Source: CAD feature listing. Evaluate the final solid. Frame: model axes, mm. A direction names the side the tool comes from. Round coordinates to 2 decimals unless told otherwise and drop trailing zeros. Order: outer loops, then holes, each group sorted by start corner. A loop starts at its lowest first (then second) coordinate and runs counter-clockwise, first axis right, second up. Notation, with made-up numbers: (18, -36.75) -> (68, -36.75) arc R14 cw to (68, -11.75) -> close; hole circle Ø4 at (-13.75, 8.5). An arc over 180 degrees is marked (long way). One line per item, written item: value. Start each with the question number.
1) Section C-C (z = 0). Return the cut outline in (x, y).
2) Reachability of faces 5 (the face through (-7.5, 0, 0)), 6 (the face through (-5, 2.25, 1)), 7 (the face through (20, 0, -19)) from +Z, -Z, +X, -X, +Y, -Y: full face, straight path, thin tool, end or side. Return the list, or none.
3) Section B-B (x = 0). Return the cut outline in (y, z), and give its area (3 significant figures).
4) Ray query, L1, parallel to X at y = -3, z = -3.25; L2, parallel to Z at x = 0, y = 4.85; L3, parallel to X at y = -2, z = -8. Return the intervals inside material, ascending.
5) Section A-A (y = -5). Return the cut outline in (x, z), and give its area (3 significant figures).
6) Mould query, pull axis X, two halves, no side actions, for faces 1 (the face through (-5, -2.25, 1)), 2 (the face through (-6.2, 0.1, 3)), 3 (the face through (0, 0, 5)), 4 (the face through (-20, 0, -19)). Classes: pulls with the +X half, pulls with the -X half, needs draft (parallel to the pull), parting line crosses it, or undercut.
7) Section D-D (y = 1). Return the cut outline in (x, z).
8) Pin query (flat end, axial travel): P1, Ø9, axis at x = 0, z = 0, coming from the -Y side; P2, Ø1.8, axis at y = 2, z = -10.5, coming from the -X side; P3, Ø5, axis at y = -4.5, z = 2, coming from the -X side; P4, Ø6.5, axis at y = 3, z = -10.5, coming from the +X side. Return the tip coordinate at first contact, or that it passes through.
```python
from build123d import *

# Parameters (mm, degrees)
SKETCH1_R                = 4
BOSS_EXTRUDE1_DEPTH      = 6
BOSS_EXTRUDE1_DEPTH_BACK = 6
CUT_EXTRUDE1_REACH       = 25
SKETCH2_W                = 1.5
SKETCH2_H                = 4.5


with BuildPart() as part:
    # Sketch1 → Boss-Extrude1 (new body, two sides)
    with BuildSketch(Plane(origin=(0, 0, 0), x_dir=(1, 0, 0), z_dir=(0, 1, 0))) as boss_extrude1_sk:
        with BuildLine():
            Line((-7.5, 3), (-7.5, -3))
            Line((-7.5, -3), (-4, -3))
            ThreePointArc((-4, -3), (-0.01892542, -4.999964183), (3.977175044, -3.030194493))
            Line((3.977175044, -3.030194493), (20, 18))
            Line((20, 18), (20, 20))
            Line((20, 20), (-20, 20))
            Line((-20, 20), (-20, 18))
            Line((-20, 18), (-7.5, 3))
        make_face()
        Circle(SKETCH1_R, mode=Mode.SUBTRACT)
        with BuildLine():
            Line((-18.047437581, 18), (-1, 18))
            Line((-1, 18), (-1, 4.898979486))
            ThreePointArc((-1, 4.898979486), (-3.189184695, 3.850857175), (-4.626858427, 1.895305015))
            Line((-4.626858427, 1.895305015), (-18.047437581, 18))
        make_face(mode=Mode.SUBTRACT)
        with BuildLine():
            Line((1, 4.898979486), (1, 18))
            Line((1, 18), (18.114239399, 18))
            Line((18.114239399, 18), (4.948014241, 0.719134947))
            ThreePointArc((4.948014241, 0.719134947), (3.634899372, 3.433293835), (1, 4.898979486))
        make_face(mode=Mode.SUBTRACT)
    extrude(amount=BOSS_EXTRUDE1_DEPTH)
    extrude(boss_extrude1_sk.sketch, amount=-BOSS_EXTRUDE1_DEPTH_BACK)

    # Sketch2 → Cut-Extrude1 (cut, up to next)
    with BuildSketch(Plane(origin=(0, 0, 3), x_dir=(-1, 0, 0), z_dir=(0, 0, -1)), mode=Mode.PRIVATE) as cut_extrude1_sk1:
        with Locations((5.15, 0)):
            Rectangle(SKETCH2_W, SKETCH2_H)
    cut_extrude1_tool1 = extrude(cut_extrude1_sk1.sketch, amount=CUT_EXTRUDE1_REACH, mode=Mode.PRIVATE) & part.part
    add(cut_extrude1_tool1.solids().sort_by_distance((-5.15, 0, 3))[0], mode=Mode.SUBTRACT)


solid = part.part
```
Findings:
1. outline: (-7.5, -6) -> (-4, -6) -> (-4, 6) -> (-7.5, 6) -> close; (4, -6) -> (6.29, -6) -> (6.29, 6) -> (4, 6) -> close; hole (-5.9, -2.25) -> (-4.4, -2.25) -> (-4.4, 2.25) -> (-5.9, 2.25) -> close
2. face 5: +Z, -X, +Y, -Y
2. face 6: +Z
2. face 7: +Z, -Z, +X, +Y, -Y
3. outline: (-6, -20) -> (6, -20) -> (6, -4) -> (-6, -4) -> close; (-6, 4) -> (6, 4) -> (6, 5) -> (-6, 5) -> close
3. area: 204 mm2
4. L1: -7.71 to -5.76, -3.8 to -2.33, 2.33 to 3.8, 6.88 to 8.76
4. L2: -20 to -4, 4 to 5
4. L3: -11.67 to -9.71, -1 to 1, 10.5 to 12.38
5. outline: (-20, -20) -> (20, -20) -> (20, -18) -> (3.98, 3.03) arc R5 ccw to (-4, 3) -> (-7.5, 3) -> (-7.5, -3) -> (-20, -18) -> close; hole (-18.05, -18) -> (-1, -18) -> (-1, -4.9) arc R5 cw to (-4.63, -1.9) -> close; hole circle Ø8 at (0, 0); hole (1, -18) -> (18.11, -18) -> (4.95, -0.72) arc R5 cw to (1, -4.9) -> close
5. area: 215 mm2
6. face 1: undercut
6. face 2: needs draft
6. face 3: parting line crosses it
6. face 4: pulls with the -X half
7. outline: (-20, -20) -> (20, -20) -> (20, -18) -> (3.98, 3.03) arc R5 ccw to (-4, 3) -> (-4.4, 3) -> (-4.4, -2.37) arc R5 ccw to (-1, -4.9) -> (-1, -18) -> (-18.05, -18) -> (-5.9, -3.42) -> (-5.9, 3) -> (-7.5, 3) -> (-7.5, -3) -> (-20, -18) -> close; hole circle Ø8 at (0, 0); hole (1, -18) -> (18.11, -18) -> (4.95, -0.72) arc R5 cw to (1, -4.9) -> close
8. P1: y = -6
8. P2: x = -14.5
8. P3: x = -7.5
8. P4: x = 16.76
